```python
from build123d import *

# Parameters (mm, degrees)
SKETCH1_W                = 94.1
SKETCH1_H                = 38.2
SKETCH1_W_2              = 91.1
SKETCH1_H_2              = 35.2
BOSS_EXTRUDE1_DEPTH      = 1
SKETCH1_3_W              = 94.1
SKETCH1_3_H              = 38.2
SKETCH1_3_W_2            = 91.1
SKETCH1_3_H_2            = 35.2
BOSS_EXTRUDE2_DEPTH      = 11
SKETCH2_W                = 1.5
SKETCH2_H                = 16
SKETCH2_H_2              = 27.5
CUT_EXTRUDE1_DEPTH       = 10
SKETCH3_W                = 8
SKETCH3_H                = 1
BOSS_EXTRUDE3_DEPTH      = 8
SKETCH4_R                = 0.5
CUT_EXTRUDE2_DEPTH       = 10
SKETCH5_R                = 1.5
BOSS_EXTRUDE4_DEPTH      = 8
SKETCH7_R                = 1.25
BOSS_EXTRUDE6_DEPTH      = 2
FILLET1_R                = 3
FILLET2_R                = 2
FILLET3_R                = 3
CHAMFER2_SIZE            = 1
SKETCH6_W                = 10
SKETCH6_H                = 0.4
BOSS_EXTRUDE5_DEPTH      = 1
FILLET4_R                = 2
CHAMFER3_SIZE            = 1
FILLET5_R                = 0.5
FILLET6_R                = 0.5
FILLET4_OF_MIRROR2_R     = 2
CHAMFER3_OF_MIRROR2_SIZE = 1


# Some blends are built 0.0001 mm under size
with BuildPart() as part:
    # Sketch1 → Boss-Extrude1 (new body)
    # profile 1 of 2: a face of its own
    with BuildSketch(Plane.XY):
        with Locations((45.55, 17.6)):
            Rectangle(SKETCH1_W, SKETCH1_H)
        with Locations((45.55, 17.6)):
            Rectangle(SKETCH1_W_2, SKETCH1_H_2, mode=Mode.SUBTRACT)
    # profile 2 of 2: a face of its own
    with BuildSketch(Plane.XY):
        with Locations((45.55, 17.6)):
            Rectangle(SKETCH1_W_2, SKETCH1_H_2)
    extrude(amount=BOSS_EXTRUDE1_DEPTH)

    # Sketch1<3> → Boss-Extrude2 (add)
    with BuildSketch(Plane.XY):
        with Locations((45.55, 17.6)):
            Rectangle(SKETCH1_3_W, SKETCH1_3_H)
        with Locations((45.55, 17.6)):
            Rectangle(SKETCH1_3_W_2, SKETCH1_3_H_2, mode=Mode.SUBTRACT)
    extrude(amount=BOSS_EXTRUDE2_DEPTH)

    # Sketch2 → Cut-Extrude1 (cut)
    with BuildSketch(Plane.XY.offset(11)):
        with Locations((-0.75, 17.6)):
            Rectangle(SKETCH2_W, SKETCH2_H)
        with Locations((91.85, 17.6)):
            Rectangle(SKETCH2_W, SKETCH2_H_2)
    extrude(amount=-CUT_EXTRUDE1_DEPTH, mode=Mode.SUBTRACT)

    # Sketch3 → Boss-Extrude3 (add)
    with BuildSketch(Plane.XY.offset(1)):
        with Locations((82.1, 31.2)):
            Rectangle(SKETCH3_W, SKETCH3_H)
        with Locations((82.1, 24.4)):
            Rectangle(SKETCH3_W, SKETCH3_H)
        with Locations((82.1, 17.6)):
            Rectangle(SKETCH3_W, SKETCH3_H)
        with Locations((82.1, 10.8)):
            Rectangle(SKETCH3_W, SKETCH3_H)
        with Locations((82.1, 4)):
            Rectangle(SKETCH3_W, SKETCH3_H)
    extrude(amount=BOSS_EXTRUDE3_DEPTH)

    # Sketch4 → Cut-Extrude2 (cut)
    with BuildSketch(Plane.XY.offset(1)):
        with Locations((84.9, 27.8)):
            Circle(SKETCH4_R)
        with Locations((84.9, 21)):
            Circle(SKETCH4_R)
        with Locations((84.9, 14.2)):
            Circle(SKETCH4_R)
        with Locations((84.9, 7.4)):
            Circle(SKETCH4_R)
    extrude(amount=-CUT_EXTRUDE2_DEPTH, mode=Mode.SUBTRACT)

    # Sketch5 → Boss-Extrude4 (add)
    with BuildSketch(Plane.XY.offset(1)):
        with Locations((4, 31)):
            Circle(SKETCH5_R)
        with Locations((4, 4.2)):
            Circle(SKETCH5_R)
    extrude(amount=BOSS_EXTRUDE4_DEPTH)

    # Sketch7 → Boss-Extrude6 (add)
    with BuildSketch(Plane.XY.offset(9)):
        with Locations((4, 31)):
            Circle(SKETCH7_R)
        with Locations((4, 4.2)):
            Circle(SKETCH7_R)
    extrude(amount=BOSS_EXTRUDE6_DEPTH)

    # Fillet1
    # the kernel refuses this fillet: 3 mm, written as the material it adds along each edge
    with BuildSketch(Plane(origin=(4, 31, 1), x_dir=(1, 0, 0), z_dir=(0, -1, 0))) as fillet1_piece_1:
        with BuildLine():
            CenterArc((1.5 + FILLET1_R, FILLET1_R), FILLET1_R, 180, 90)
            Line((1.5, FILLET1_R), (1.5, 0))
            Line((1.5, 0), (1.5 + FILLET1_R, 0))
        make_face()
    revolve(axis=Axis((4, 31, 1), (0, 0, 1)))
    with BuildSketch(Plane(origin=(4, 4.2, 1), x_dir=(1, 0, 0), z_dir=(0, -1, 0))) as fillet1_piece_2:
        with BuildLine():
            CenterArc((1.5 + FILLET1_R, FILLET1_R), FILLET1_R, 180, 90)
            Line((1.5, FILLET1_R), (1.5, 0))
            Line((1.5, 0), (1.5 + FILLET1_R, 0))
        make_face()
    revolve(axis=Axis((4, 4.2, 1), (0, 0, 1)))

    # Fillet2
    fillet2_edges = [part.edges().sort_by_distance(p)[0] for p in [
        (78.1, 17.6, 1),
        (82.1, 17.1, 1),
        (86.1, 17.6, 1),
        (82.1, 18.1, 1),
        (78.1, 10.8, 1),
        (82.1, 10.3, 1),
        (86.1, 10.8, 1),
        (82.1, 11.3, 1),
        (78.1, 4, 1),
        (82.1, 3.5, 1),
        (86.1, 4, 1),
        (82.1, 4.5, 1),
        (78.1, 31.2, 1),
        (82.1, 30.7, 1),
        (86.1, 31.2, 1),
        (82.1, 31.7, 1),
        (78.1, 24.4, 1),
        (82.1, 23.9, 1),
        (86.1, 24.4, 1),
        (82.1, 24.9, 1),
    ]]
    fillet(fillet2_edges, radius=FILLET2_R)

    # Fillet3
    fillet3_edges = [part.edges().sort_by_distance(p)[0] for p in [
        (-1.5, 36.7, 5.5),
        (92.6, 36.7, 5.5),
        (92.6, -1.5, 5.5),
        (-1.5, -1.5, 5.5),
    ]]
    fillet(fillet3_edges, radius=FILLET3_R)

    # Chamfer2
    chamfer2_edges = [part.edges().sort_by_distance(p)[0] for p in [
        (-1.5, 17.6, 0),
        (45.55, 36.7, 0),
        (92.6, 17.6, 0),
        (45.55, -1.5, 0),
        (91.721320344, -0.621320344, 0),
        (-0.621320344, -0.621320344, 0),
        (91.721320344, 35.821320344, 0),
        (-0.621320344, 35.821320344, 0),
    ]]
    chamfer(chamfer2_edges, length=CHAMFER2_SIZE - 0.0001)  # a hair under: the kernel refuses the full size

    # Sketch6 → Boss-Extrude5 (add)
    with BuildSketch(Plane.XZ.offset(-35.2)):
        with Locations((45.55, 10.8)):
            Rectangle(SKETCH6_W, SKETCH6_H)
    boss_extrude5 = extrude(amount=BOSS_EXTRUDE5_DEPTH)

    # Fillet4
    # the kernel refuses this fillet: 2 mm, written as the material it adds along each edge
    with BuildSketch(Plane(origin=(40.55, 35.2, 10.6), x_dir=(-1, 0, 0), z_dir=(0, 0, 1)), Plane(origin=(50.55, 35.2, 11), x_dir=(1, 0, 0), z_dir=(0, 0, -1))) as fillet4_piece_1:
        with BuildLine():
            CenterArc((1.732050808, 2), FILLET4_R, 210, 60)
            Line((0, 1), (-0.034641016, 0.98))
            ThreePointArc((-0.034641016, 0.98), (-0.04, 0.5), (-0.04, 0))
            Line((-0.04, 0), (0, -0.04))
            Line((0, -0.04), (1.732050808, -0.04))
            Line((1.732050808, -0.04), (1.732050808, 0))
        make_face()
    extrude(amount=0.4)

    # Chamfer3
    # the kernel refuses this chamfer: 1 mm, written as the material it takes off along each edge
    with BuildSketch(Plane(origin=(37.978317012, 34.2, 11), x_dir=(0, 0.9996219169112968, 0.02749587661058555), z_dir=(1, 0, 0))) as chamfer3_piece_1:
        Polygon((CHAMFER3_SIZE * 0.999621916911, -CHAMFER3_SIZE * 0.0274958766106), (-CHAMFER3_SIZE * 0.0274958766106, -CHAMFER3_SIZE * 0.999621916911), (0, 0), align=None)
    extrude(amount=15.143365976, mode=Mode.SUBTRACT)

    # Fillet5
    # the kernel refuses this fillet: 0.5 mm, written as the material it adds along each edge
    with BuildSketch(Plane(origin=(4, 31, 9), x_dir=(1, 0, 0), z_dir=(0, -1, 0))) as fillet5_piece_1:
        with BuildLine():
            CenterArc((1.75, 0.433012702), FILLET5_R, 180, 60)
            Line((1.25, 0.433012702), (1.24, 0.433012702))
            Line((1.24, 0.433012702), (1.24, 0))
            Line((1.24, 0), (1.25, -0.01))
            ThreePointArc((1.25, -0.01), (1.375, -0.01), (1.495, -0.008660254))
            Line((1.495, -0.008660254), (1.5, 0))
        make_face()
    revolve(axis=Axis((4, 31, 9), (0, 0, 1)))
    with BuildSketch(Plane(origin=(4, 4.2, 9), x_dir=(1, 0, 0), z_dir=(0, -1, 0))) as fillet5_piece_2:
        with BuildLine():
            CenterArc((1.75, 0.433012702), FILLET5_R, 180, 60)
            Line((1.25, 0.433012702), (1.24, 0.433012702))
            Line((1.24, 0.433012702), (1.24, 0))
            Line((1.24, 0), (1.25, -0.01))
            ThreePointArc((1.25, -0.01), (1.375, -0.01), (1.495, -0.008660254))
            Line((1.495, -0.008660254), (1.5, 0))
        make_face()
    revolve(axis=Axis((4, 4.2, 9), (0, 0, 1)))

    # Fillet6
    fillet6_edges = [part.edges().sort_by_distance(p)[0] for p in [
        (2.5, 31, 9),
        (2.5, 4.2, 9),
    ]]
    fillet(fillet6_edges, radius=FILLET6_R)

    # Mirror2: Boss-Extrude5 across plane
    add(boss_extrude5.mirror(Plane(origin=(0, 17.6, 0), x_dir=(0, 0, 1), z_dir=(0, -1, 0))))

    # Fillet4 of Mirror2
    # the kernel refuses this fillet: 2 mm, written as the material it adds along each edge
    with BuildSketch(Plane(origin=(40.55, 0, 10.6), x_dir=(-1, 0, 0), z_dir=(0, 0, 1)), Plane(origin=(50.55, 0, 11), x_dir=(1, 0, 0), z_dir=(0, 0, -1))) as fillet4_of_mirror2_piece_1:
        with BuildLine():
            CenterArc((1.732050808, -2), FILLET4_OF_MIRROR2_R, 90, 60)
            Line((0, -1), (-0.034641016, -0.98))
            ThreePointArc((-0.034641016, -0.98), (-0.04, -0.5), (-0.04, 0))
            Line((-0.04, 0), (0, 0.04))
            Line((0, 0.04), (1.732050808, 0.04))
            Line((1.732050808, 0.04), (1.732050808, 0))
        make_face()
    extrude(amount=0.4)

    # Chamfer3 of Mirror2
    # the kernel refuses this chamfer: 1 mm, written as the material it takes off along each edge
    with BuildSketch(Plane(origin=(37.978317012, 1, 11), x_dir=(0, -0.9996219169112968, 0.02749587661058563), z_dir=(1, 0, 0))) as chamfer3_of_mirror2_piece_1:
        Polygon((CHAMFER3_OF_MIRROR2_SIZE * 0.999621916911, CHAMFER3_OF_MIRROR2_SIZE * 0.0274958766106), (-CHAMFER3_OF_MIRROR2_SIZE * 0.0274958766106, CHAMFER3_OF_MIRROR2_SIZE * 0.999621916911), (0, 0), align=None)
    extrude(amount=15.143365976, mode=Mode.SUBTRACT)


solid = part.part
```
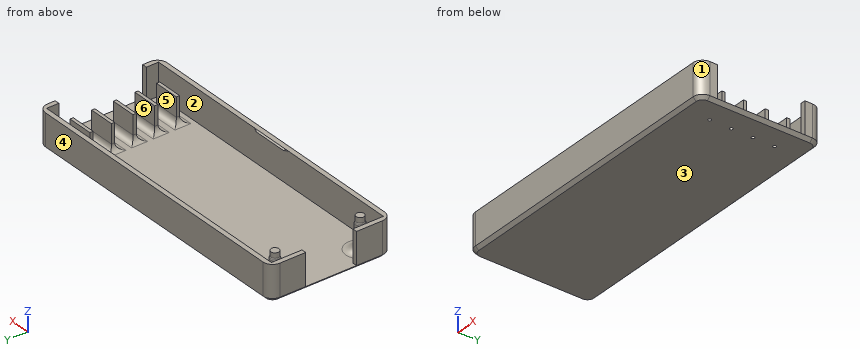
Check sheet for the modelled part. Datum: model origin and axes. Units: mm. Face numbers are marked on the shaded views. A direction names the side the tool comes from. Round coordinates to 2 decimals unless told otherwise and drop trailing zeros. Order: outer loops, then holes, each group sorted by start corner. A loop starts at its lowest first (then second) coordinate and runs counter-clockwise, first axis right, second up.
1) Section check A-A (x = 13.5). Record the boundary of the cut face in (y, z), and give its area (3 significant figures).
2) Scan lines: line 1 (Y direction, x = 64, z = 4); line 2 (Y direction, x = 84.9, z = 0.45); line 3 (Y direction, x = 84.9, z = 0.55). Record each from-to range of solid material in increasing order.
3) Tool access check on the marked faces 4, 5 and 6. Record the directions out of +Z, -Z, +X, -X, +Y, -Y that give a thin tool (end or side, any length) a straight path to the whole face; none if there is none.
4) Go/stop test with flat-tipped pins: pin 1 Ø1.2 at (x, z) = (-0.5, 6) entering from -Y; pin 2 Ø10 at (x, y) = (76.5, 24) entering from +Z; pin 3 Ø3 at (y, z) = (4, 7) entering from +X; pin 4 Ø1.5 at (y, z) = (18, 9) entering from +X. Record where each tip stops, or that it passes through.
5) Section check B-B (z = 5.75). Give the number of separate pieces and of enclosed holes in the cut face, and give its area (3 significant figures).
6) Mould release check, pull along X, two halves, no side actions. Record for the marked faces 1, 2 and 3: +X half, -X half, draft (parallel to the pull), parting line (faces both ways), or undercut.
Result:
1. outline: (-1.5, 1) - (-0.5, 0) - (35.7, 0) - (36.7, 1) - (36.7, 11) - (35.2, 11) - (35.2, 1) - (0, 1) - (0, 11) - (-1.5, 11) - close
1. area: 67.2 mm2
2. line 1: y = -1.5 to 0, 35.2 to 36.7
2. line 2: y = -0.95 to 6.9, 7.9 to 13.7, 14.7 to 20.5, 21.5 to 27.3, 28.3 to 36.15
2. line 3: y = -1.05 to 6.9, 7.9 to 13.7, 14.7 to 20.5, 21.5 to 27.3, 28.3 to 36.25
3. face 4: +Z, -Z, +X, -X, +Y
3. face 5: +Z, +X
3. face 6: +Z, +X, -X
4. pin 1: stops at y = -1.15
4. pin 2: stops at z = 9
4. pin 3: stops at x = 92.6
4. pin 4: stops at x = 86.1
5. separate pieces: 9
5. enclosed holes: 0
5. area: 369 mm2
6. face 1: +X half
6. face 2: undercut
6. face 3: draft
